For this review, take the finished solid that the model builds, in its own axes (mm). A direction names the side the tool comes from. Round coordinates to 2 decimals unless told otherwise and drop trailing zeros. Write each loop counter-clockwise with the first axis right and the second up, starting at its lowest first coordinate (ties: lowest second). Pieces come first, ordered by that corner, then holes.
from build123d import *

# Parameters (mm, degrees)
SKETCH_W              = 56.3
SKETCH_H              = 78
PAD_DEPTH             = 28.15
PAD_DEPTH_BACK        = 28.15
POCKET_DEPTH          = 73.2
POLARPATTERN_COUNT    = 4
SKETCH002_R           = 2.6
POCKET001_DEPTH       = 5
POLARPATTERN001_COUNT = 4
SKETCH003_R           = 19.05
PAD001_DEPTH          = 1.6
SKETCH004_R           = 5
POCKET002_DEPTH       = 2
SKETCH005_R           = 5
POCKET003_DEPTH       = 2
SKETCH006_R           = 3.175
PAD002_DEPTH          = 100


with BuildPart() as part:
    # Sketch → Pad (new body, two sides)
    with BuildSketch(Plane.XY) as pad_sk:
        with Locations((0, 39)):
            Rectangle(SKETCH_W, SKETCH_H)
    extrude(amount=PAD_DEPTH)
    extrude(pad_sk.sketch, amount=-PAD_DEPTH_BACK)

    # Sketch001 → Pocket (cut)
    with BuildSketch(Plane.XZ):
        with BuildLine():
            Line((18.15, 28.15), (28.15, 28.15))
            Line((28.15, 28.15), (28.15, 18.15))
            Line((28.15, 18.15), (24.007864, 18.15))
            ThreePointArc((18.15, 24.007864), (19.865729, 19.865729), (24.007864, 18.15))
            Line((18.15, 24.007864), (18.15, 28.15))
        make_face()
    pocket = extrude(amount=-POCKET_DEPTH, mode=Mode.SUBTRACT)

    # PolarPattern: Pocket ×4 about axis
    polarpattern_axis = Axis((0, 0, 0), (0, -1, 0))
    for i in range(1, POLARPATTERN_COUNT):
        add(pocket.rotate(polarpattern_axis, i * 360 / POLARPATTERN_COUNT), mode=Mode.SUBTRACT)

    # Sketch002 → Pocket001 (cut)
    with BuildSketch(Plane(origin=(0, 78, 0), x_dir=(-1, 0, 0), z_dir=(0, 1, 0))):
        with Locations((23.55, 23.55)):
            Circle(SKETCH002_R)
    pocket001 = extrude(amount=-POCKET001_DEPTH, mode=Mode.SUBTRACT)

    # PolarPattern001: Pocket001 ×4 about axis
    polarpattern001_axis = Axis((0, 78, 0), (0, 1, 0))
    for i in range(1, POLARPATTERN001_COUNT):
        add(pocket001.rotate(polarpattern001_axis, i * 360 / POLARPATTERN001_COUNT), mode=Mode.SUBTRACT)

    # Sketch003 → Pad001 (new body)
    with BuildSketch(Plane(origin=(0, 78, 0), x_dir=(-1, 0, 0), z_dir=(0, 1, 0))):
        Circle(SKETCH003_R)
    extrude(amount=PAD001_DEPTH)

    # Sketch004 → Pocket002 (cut)
    with BuildSketch(Plane(origin=(0, 79.6, 0), x_dir=(-1, 0, 0), z_dir=(0, 1, 0))):
        Circle(SKETCH004_R)
    extrude(amount=-POCKET002_DEPTH, mode=Mode.SUBTRACT)

    # Sketch005 → Pocket003 (cut)
    with BuildSketch(Plane.XZ):
        Circle(SKETCH005_R)
    extrude(amount=-POCKET003_DEPTH, mode=Mode.SUBTRACT)

    # Sketch006 → Pad002 (new body)
    with BuildSketch(Plane.XZ.offset(-2)):
        Circle(SKETCH006_R)
    extrude(amount=-PAD002_DEPTH)


solid = part.part
(1) For faces 1 (the face through (-1, 77.6, -3.3)), 2 (the face through (-26, 36, -18.15)), 3 (the face through (22, 73.2, 21)), list the 3-axis set-ups (+Z, -Z, +X, -X, +Y, -Y) from which the entire face can be reached by the end or side of a thin tool; tool diameter is ignored.
Geometry check:
face 1: +Y
face 2: -Z, -X, -Y
face 3: +Z, +X, -Y
(2) We need section B-B, the plane y = 11. Give the boundary of the cut face in (x, z).
Geometry check:
outline: (-28.15, -18.15) - (-24.01, -18.15) arc R5.86 cw to (-18.15, -24.01) - (-18.15, -28.15) - (18.15, -28.15) - (18.15, -24.01) arc R5.86 cw to (24.01, -18.15) - (28.15, -18.15) - (28.15, 18.15) - (24.01, 18.15) arc R5.86 cw to (18.15, 24.01) - (18.15, 28.15) - (-18.15, 28.15) - (-18.15, 24.01) arc R5.86 cw to (-24.01, 18.15) - (-28.15, 18.15) - close
(3) We need section D-D, the plane z = 6.5. Give the boundary of the cut face in (x, y), and give its area (3 significant figures).
Geometry check:
outline: (-28.15, 0) - (28.15, 0) - (28.15, 78) - (17.91, 78) - (17.91, 79.6) - (-17.91, 79.6) - (-17.91, 78) - (-28.15, 78) - close
area: 4,450 mm2
(4) Mouldability with a two-part tool opening along X and no side actions: class faces 4 (the face through (0, 40, -28.15)), 5 (the face through (19.91, 36.09, -19.82)), 6 (the face through (-1.08, 0.99, -4.88)) as pulls with the +X half, pulls with the -X half, needs draft (parallel to the pull), parting line crosses it, or undercut.
Geometry check:
face 4: needs draft
face 5: pulls with the +X half
face 6: undercut
(5) We need section A-A, the plane y = 74.5. Give the boundary of the cut face in (x, z), and give its area (3 significant figures).
Geometry check:
outline: (-28.15, -28.15) - (28.15, -28.15) - (28.15, 28.15) - (-28.15, 28.15) - close; hole circle Ø5.2 at (-23.55, -23.55); hole circle Ø5.2 at (-23.55, 23.55); hole circle Ø5.2 at (23.55, -23.55); hole circle Ø5.2 at (23.55, 23.55)
area: 3,080 mm2
(6) We need section C-C, the plane x = 0. Give the boundary of the cut face in (y, z) (3 decimals).
Geometry check:
outline: (0, -28.15) - (78, -28.15) - (78, -19.05) - (79.6, -19.05) - (79.6, -5) - (77.6, -5) - (77.6, -3.175) - (102, -3.175) - (102, 3.175) - (77.6, 3.175) - (77.6, 5) - (79.6, 5) - (79.6, 19.05) - (78, 19.05) - (78, 28.15) - (0, 28.15) - (0, 5) - (2, 5) - (2, -5) - (0, -5) - close
(7) For line 1 along Z through (x, y) = (0, 78.1) (3 decimals); line 2 along Y through (x, z) = (7, -21.5); line 3 along Y through (x, z) = (0.5, -19), list the stretches that pass through material, from the lowest coordinate up.
Geometry check:
line 1: z = -19.05 to -5, -3.175 to 3.175, 5 to 19.05
line 2: y = 0 to 78
line 3: y = 0 to 79.6
(8) For pin 1 Ø2 at (x, y) = (-26, 54) entering from +Z; pin 2 Ø4.5 at (y, z) = (44, -27) entering from -X; pin 3 Ø1.5 at (x, z) = (-19, -7.5) entering from +Y, all flat-tipped, find the tip position at first contact; note any pin that passes through.
Geometry check:
pin 1: stops at z = 18.15
pin 2: stops at x = -18.15
pin 3: stops at y = 78
